Model file for the job. Use its own axes, mm. Face numbers are marked on the shaded views. A direction names the side the tool comes from. Round coordinates to 2 decimals unless told otherwise and drop trailing zeros. Loops run counter-clockwise (first coordinate to the right, second up) from the corner with the lowest first, then second, coordinate; pieces in that order, holes last. Notation, with made-up numbers: (14, 66.25) - (54, 66.25) arc R18 cw to (54, 79.25) - close; hole circle Ø10 at (41, 77.5). An arc over 180 degrees is marked (long way). Answer as a JSON object with one key per item and string values.
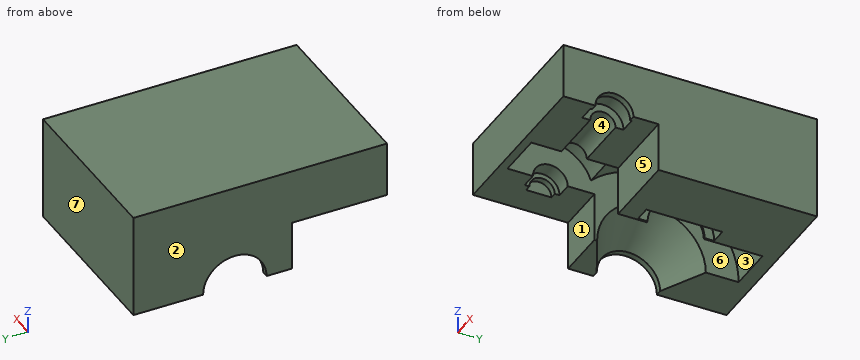
Solid Edge part; units mm, degrees
sketch "Sketch1" plane through (0, 0, 0) normal (0, 0, 1) x (1, 0, 0)
  line L0 (-28, -40) -> (28, -40)
  line L1 (28, -40) -> (28, 40)
  line L2 (28, 40) -> (-28, 40)
  line L3 (-28, 40) -> (-28, -40)
  dimension "D1" = 28
  dimension "D2" = 28
extrude "Protrusion1" add sketch "Sketch1" along normal blind 60
sketch "Sketch2" plane through (8, 0, 21.28) normal (-1, 0, 0) x (0, -1, 0)
  circle A0 centre (-8, 5.72) radius 12
extrude "Extrusionsausschnitt_3" cut sketch "Sketch2" along normal blind 5
sketch "Sketch3" plane through (3, 5.5, 20.5) normal (1, 0, 0) x (0, 1, 0)
  circle A0 centre (2.5, 6.5) radius 9
extrude "Extrusionsausschnitt_4" cut sketch "Sketch3" against normal blind 1.5
sketch "Sketch4" plane through (1.5, 5.5, 22.5) normal (1, 0, 0) x (0, 1, 0)
  circle A0 centre (2.5, 4.5) radius 27.5
extrude "Extrusionsausschnitt_5" cut sketch "Sketch4" against normal blind 13.5
sketch "Sketch5" plane through (1.5, 5.5, 21.28) normal (-1, 0, 0) x (0, 0, 1)
  circle A0 centre (5.72, 2.5) radius 27.5
extrude "Extrusionsausschnitt_6" cut sketch "Sketch5" against normal blind 1
sketch "Sketch6" plane through (0, 15, 27) normal (0, 0, 1) x (1, 0, 0)
  line L0 (-12, 10.1524) -> (-28, 2)
  line L1 (-12, 10.1524) -> (-12, -7)
revolve "RevolvedCutout1" cut sketch "Sketch6" angle 360 about axis through (-28, 8, 27) along (1, 0, 0) material side at (-19.9773, 21.0316, 27)
sketch "Sketch7" plane through (-28, 0, 21.28) normal (-1, 0, 0) x (0, -1, 0)
  circle A0 centre (-8, 5.72) radius 10
extrude "Cutout1" cut sketch "Sketch7" against normal up to vertex (16 mm away)
sketch "Sketch8" plane through (-12, 0, 21.28) normal (-1, 0, 0) x (0, 0, 1)
  circle A0 centre (21.28, -23.91) radius 13.5
  dimension "D1" = 21.28
extrude "Extrusionsausschnitt_8" cut sketch "Sketch8" against normal up to vertex (14.5 mm away)
sketch "Sketch9" plane through (-12, -0.75, 21.28) normal (1, 0, 0) x (0, 1, 0)
  circle A0 centre (-23.16, 21.28) radius 5.5
extrude "Extrusionsausschnitt_9" cut sketch "Sketch9" against normal blind 5
sketch "Sketch10" plane through (-17, -23.91, 39.81) normal (1, 0, 0) x (0, 1, 0)
  circle A0 centre (0, 2.75) radius 4
extrude "Extrusionsausschnitt_10" cut sketch "Sketch10" against normal blind 2
sketch "Sketch11" plane through (2.5, -0.75, 21.28) normal (-1, 0, 0) x (0, -1, 0)
  circle A0 centre (23.16, 21.28) radius 4
extrude "Extrusionsausschnitt_11" cut sketch "Sketch11" against normal blind 17.5
sketch "Sketch12" plane through (20, -23.91, 40.56) normal (-1, 0, 0) x (0, -1, 0)
  circle A0 centre (0, 2) radius 6.5
extrude "Extrusionsausschnitt_12" cut sketch "Sketch12" against normal blind 5
sketch "Sketch13" plane through (25, -23.91, 38.81) normal (-1, 0, 0) x (0, -1, 0)
  circle A0 centre (0, 3.75) radius 6
extrude "Extrusionsausschnitt_13" cut sketch "Sketch13" against normal blind 24
sketch "Sketch14" plane through (28, 0, 21.28) normal (1, 0, 0) x (0, 1, 0)
  circle A0 centre (-23.6974, 21.295) radius 9.5
extrude "Extrusionsausschnitt_14" cut sketch "Sketch14" against normal blind 1
sketch "Sketch15" plane through (15.25, -14.955, 42.56) normal (0, 0, 1) x (1, 0, 0)
  line L0 (11.75, 54.955) -> (11.75, -25.045)
extrude "Extrusionsausschnitt_15" cut sketch "Sketch15" along normal mid plane 96 material side at (27.05, 0, 42.56)
sketch "Sketch16" plane through (27, 0, 30) normal (1, 0, 0) x (0, 1, 0)
  line L0 (40, -3) -> (-10, -3)
  line L1 (-10, -3) -> (-10, 12.56)
  line L2 (-10, 12.56) -> (-40, 12.56)
extrude "Extrusionsausschnitt_16" cut sketch "Sketch16" against normal blind 80 material side at (27, 15, 26.95)
properties material "Aluminiumlegierung:3.0205, Al 99.0, EN-AW 1200"
1) Slice it at A-A on y = -23.91. List the corners of the cut face in (x, z).
Values follow:
{"outline": "(-28, 42.56) - (-19, 42.56) - (-19, 46.56) - (-17, 46.56) - (-17, 48.06) - (-12, 48.06) - (-12, 56.06) - (2.5, 56.06) - (2.5, 46.56) - (20, 46.56) - (20, 49.06) - (25, 49.06) - (25, 48.56) - (27, 48.56) - (27, 60) - (-28, 60) - close"}
2) Probe probe 1 along X at (y, z) = (28.5, 36); probe 2 along Y at (x, z) = (-5, 52.5); probe 3 along Y at (x, z) = (22.5, 46.5). List the from-to ranges inside material, lowest first.
Values follow:
{"probe 1": "-28 to -12, 2.5 to 27", "probe 2": "-40 to -33.04, -14.78 to -2.3, 18.3 to 40", "probe 3": "-40 to -29.08, -18.74 to 40"}
3) Slice it at C-C on y = 8. List the corners of the cut face in (x, z).
Values follow:
{"outline": "(-28, 37) - (-26.04, 37) - (-12, 44.15) - (-12, 54.5) - (2.5, 54.5) - (2.5, 36) - (3, 36) - (3, 39) - (8, 39) - (8, 27) - (27, 27) - (27, 60) - (-28, 60) - close"}
4) Drop flat-ended pins along their axis: P1, Ø6, axis at x = 8, z = 42, coming from the -Y side; P2, Ø3, axis at y = -25, z = 44, coming from the +X side; P3, Ø17, axis at x = 13.5, z = 31.5, coming from the -Y side; P4, Ø15, axis at x = 4, y = -22.5, coming from the -Z side. Give the stop position or say it passes through.
Values follow:
{"P1": "y = -40", "P2": "x = -19", "P3": "y = -10", "P4": "z = 42.56"}
5) Tool access for the marked faces 4, 5, 6 and 7: list every direction of +Z, -Z, +X, -X, +Y, -Y with a clear straight run to the whole face (end or side of a thin tool).
Values follow:
{"face 4": "-Z, +X", "face 5": "-Z, +X, -X, -Y", "face 6": "-Z", "face 7": "+Z, -Z, +X, -X, +Y"}
6) Slice it at D-D on z = 45.5. List the corners of the cut face in (x, y).
Values follow:
{"outline": "(-28, -40) - (27, -40) - (27, -29.14) - (25, -29.14) - (25, -29.71) - (20, -29.71) - (20, -26.62) - (2.5, -26.62) - (2.5, -37.09) - (-12, -37.09) - (-12, -28.56) - (-17, -28.56) - (-17, -26.62) - (-19, -26.62) - (-19, -21.2) - (-17, -21.2) - (-17, -19.26) - (-12, -19.26) - (-12, 28.35) - (2.5, 28.35) - (2.5, -21.2) - (20, -21.2) - (20, -18.11) - (25, -18.11) - (25, -18.68) - (27, -18.68) - (27, 40) - (-28, 40) - close"}
7) Two-plate mould, pull along Y, no slides. Class the marked faces 1, 2 and 3: pulls with the +Y half, pulls with the -Y half, needs draft (parallel to the pull), parting line crosses it, or undercut.
Values follow:
{"face 1": "pulls with the -Y half", "face 2": "needs draft", "face 3": "undercut"}
8) Slice it at B-B on x = 18. List the corners of the cut face in (y, z), then the cut area to 3 significant figures.
Values follow:
{"outline": "(-40, 42.56) - (-27.91, 42.56) arc R4 cw to (-19.91, 42.56) - (-10, 42.56) - (-10, 27) - (40, 27) - (40, 60) - (-40, 60) - close", "area": "2,150 mm²"}
